Source: CAD feature listing. Evaluate the final solid. Frame: model axes, mm. A direction names the side the tool comes from. Coordinates: 2 decimals unless noted, no trailing zeros. Write each loop counter-clockwise with the first axis right and the second up, starting at its lowest first coordinate (ties: lowest second). Pieces come first, ordered by that corner, then holes. Notation, with made-up numbers: (3.25, 71.5) - (25.25, 71.5) arc R15 cw to (25.25, 84.5) - close; hole circle Ø5 at (17, 1.5). An arc over 180 degrees is marked (long way). One line per question, with ' | ' between items. Start each with the question number.
Q1. Draft query along X for faces 3 (the face through (0, 117, 0)), 4 (the face through (-2.17, -72.26, 9.86)), 5 (the face through (25, 115, 10)), 6 (the face through (-1.3, 292.9, -44.4)). Return one class per face: +X half, -X half, draft (parallel to the pull), parting line (faces both ways), or undercut.
Q2. Contact query for flat-ended pins moving along their axis: P1, Ø12, axis at x = 7, z = -66.5, coming from the +Y side; P2, Ø1.5, axis at x = -19, y = 151, coming from the +Z side; P3, Ø6, axis at x = -20, y = -2, coming from the +Z side. Output: stop coordinate, or through.
Q3. Cut plane A-A, the plane x = 0. Return loops of the section in (y, z).
Q4. Access query for faces 1 (the face through (0, 327.5, 13)), 2 (the face through (0, 37.5, 23)). Directions: +Z, -Z, +X, -X, +Y, -Y. A direction counts if a zero-diameter tool reaches every point of the face in a straight line with its end or side. Return the directions, or none.
Q5. Line query: line 1 (X direction, y = -62, z = 9); line 2 (Y direction, x = 0, z = 14); line 3 (Z direction, x = -22, y = -0.5). Output: solid intervals per line, ascending.
Q6. Cut plane B-B, the plane y = -62.5. Return loops of the section in (x, z), plus the area to 3 significant figures.
Q7. Cut plane C-C, the plane y = 81. Return loops of the section in (x, z).
Q8. Cut plane D-D, the plane z = -75.5. Return loops of the section in (x, y), plus the area to 3 significant figures.
```python
from build123d import *

# Parameters (mm, degrees)
ESQUISSE1_W        = 50
ESQUISSE1_H        = 125
ESQUISSE1_R        = 10
BOSS_EXTRU_1_DEPTH = 20
BOSS_EXTRU_2_DEPTH = 290
ESQUISSE4_R        = 10
BOSS_EXTRU_3_DEPTH = 90
CONG_1_R           = 10


with BuildPart() as part:
    # Esquisse1 → Boss.-Extru.1 (new body)
    with BuildSketch(Plane.XY):
        with Locations((0, -25)):
            Rectangle(ESQUISSE1_W, ESQUISSE1_H)
        with Locations((0, -62.5)):
            Circle(ESQUISSE1_R, mode=Mode.SUBTRACT)
    extrude(amount=BOSS_EXTRU_1_DEPTH)

    # Esquisse2 → Boss.-Extru.2 (add)
    with BuildSketch(Plane(origin=(0, 37.5, 0), x_dir=(1, 0, 0), z_dir=(0, 1, 0))):
        with BuildLine():
            ThreePointArc((25, -0.81456696), (24.846070853, -0.405994408), (24.685464957, 0))
            Line((24.685464957, 0), (-24.685464957, 0))
            ThreePointArc((-24.685464957, 0), (-24.846070853, -0.405994408), (-25, -0.81456696))
            Line((-25, -0.81456696), (-25, -19.18543304))
            ThreePointArc((-25, -19.18543304), (0, -36.634041753), (25, -19.18543304))
            Line((25, -19.18543304), (25, -0.81456696))
        make_face()
    extrude(amount=BOSS_EXTRU_2_DEPTH)

    # Esquisse4 → Boss.-Extru.3 (add)
    with BuildSketch(Plane(origin=(0, 0, 0), x_dir=(-1, 0, 0), z_dir=(0, 0, -1))):
        with Locations(Location((0, 302.814535043, 0), (0, 0, 180))):
            Circle(ESQUISSE4_R)
    extrude(amount=BOSS_EXTRU_3_DEPTH)

    # Congé1
    # the kernel refuses this fillet: 10 mm, written as the material it takes off along each edge
    with BuildSketch(Plane(origin=(0, 37.5, 10), x_dir=(-0.8501027120778188, 0, -0.5266169185640897), z_dir=(0.5266169185640897, 0, -0.8501027120778188))) as cong_1_piece_1_section:
        with BuildLine():
            CenterArc((26.634041753 - CONG_1_R, CONG_1_R), CONG_1_R, 270, 90)
            Line((26.634041753 - CONG_1_R, 0), (26.634041753, 0))
            Line((26.634041753, 0), (26.634041753, CONG_1_R))
        make_face()
    cong_1_piece_1 = revolve(axis=Axis((0, 37.5, 10), (0, 1, 0)), revolution_arc=243.554314658, mode=Mode.PRIVATE)
    cong_1_piece_1 = split(cong_1_piece_1, bisect_by=Plane(origin=(0, 40.353738925, 20), z_dir=(0, 0, 1)), keep=Keep.TOP, mode=Mode.PRIVATE)
    add(cong_1_piece_1, mode=Mode.SUBTRACT)
    with BuildSketch(Plane(origin=(0, 327.5, 10), x_dir=(-0.8323565470530717, 0, -0.5542405421636779), z_dir=(0.5542405421636779, 0, -0.8323565470530717))) as cong_1_piece_2:
        with BuildLine():
            CenterArc((26.634041753 - CONG_1_R, -CONG_1_R), CONG_1_R, 0, 90)
            Line((26.634041753, -CONG_1_R), (26.634041753, 0))
            Line((26.634041753, 0), (26.634041753 - CONG_1_R, 0))
        make_face()
    revolve(axis=Axis((0, 327.5, 10), (0, 1, 0)), revolution_arc=247.316842265, mode=Mode.SUBTRACT)
    with BuildSketch(Plane(origin=(0, 327.5, 10), x_dir=(0.8328594865150245, 0, 0.5534844855295674), z_dir=(-0.5534844855295674, 0, 0.8328594865150245))) as cong_1_piece_3:
        with BuildLine():
            CenterArc((26.634041753 - CONG_1_R, -CONG_1_R), CONG_1_R, 0, 90)
            Line((26.634041753, -CONG_1_R), (26.634041753, 0))
            Line((26.634041753, 0), (26.634041753 - CONG_1_R, 0))
        make_face()
    revolve(axis=Axis((0, 327.5, 10), (0, 1, 0)), revolution_arc=109.439699246, mode=Mode.SUBTRACT)
    with BuildSketch(Plane(origin=(0, 327.5, 10), x_dir=(-0.2447438061673637, 0, -0.9695877832061993), z_dir=(0.9695877832061993, 0, -0.2447438061673637))) as cong_1_piece_4:
        with BuildLine():
            CenterArc((26.634041753 - CONG_1_R, -CONG_1_R), CONG_1_R, 0, 90)
            Line((26.634041753 - CONG_1_R, 0), (26.634041753, 0))
            Line((26.634041753, 0), (26.634041753, -CONG_1_R))
        make_face()
    revolve(axis=Axis((0, 327.5, 10), (0, 1, 0)), revolution_arc=109.439699247, mode=Mode.SUBTRACT)


solid = part.part
```
Reply:
1) face 3: draft | face 4: undercut | face 5: +X half | face 6: parting line
2) P1: stops at y = 312.76 | P2: stops at z = 29.4 | P3: stops at z = 20
3) outline: (-87.5, 0) - (-72.5, 0) - (-72.5, 20) - (-87.5, 20) - close; (-52.5, 0) - (292.81, 0) - (292.81, -90) - (312.81, -90) - (312.81, 0) - (327.5, 0) - (327.5, 26.63) arc R10 ccw to (317.5, 36.63) - (47.5, 36.63) arc R10 ccw to (37.5, 26.63) - (37.5, 20) - (-52.5, 20) - close
4) face 1: +Z, -Z, +X, -X, +Y | face 2: +Z, +X, -X, -Y
5) line 1: x = -25 to -9.99, 9.99 to 25 | line 2: y = -87.5 to -72.5, -52.5 to 327.5 | line 3: z = 0 to 20
6) outline: (-25, 0) - (-10, 0) - (-10, 20) - (-25, 20) - close; (10, 0) - (25, 0) - (25, 20) - (10, 20) - close | area: 600 mm^2
7) outline: (-25, 0.81) arc R26.63 ccw to (-24.69, 0) - (24.69, 0) arc R26.63 ccw to (25, 0.81) - (25, 19.19) arc R26.63 ccw to (-25, 19.19) - close
8) outline: circle Ø20 at (0, 302.81) | area: 314 mm^2
